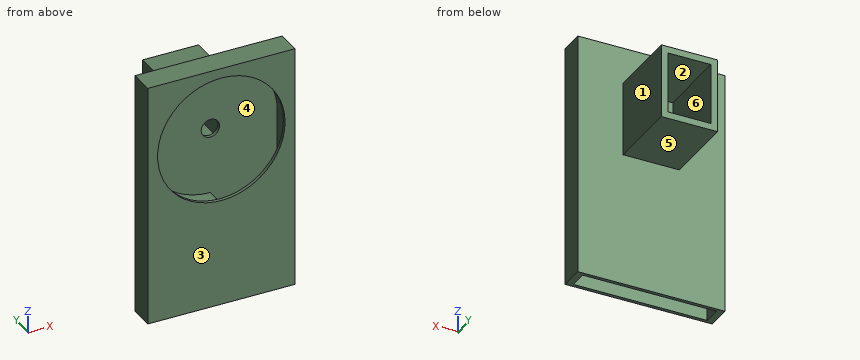
Autodesk Inventor part; units mm, degrees
ref_plane "YZ Plane" through (0, 0, 0) normal (1, 0, 0) x (0, 1, 0)
ref_plane "XZ Plane" through (0, 0, 0) normal (0, 1, 0) x (-1, 0, 0)
ref_plane "XY Plane" through (0, 0, 0) normal (0, 0, 1) x (1, 0, 0)
sketch "Sketch1" plane through (0, 0, 0) normal (0, 0, 1) x (1, 0, 0)
  line L0 (0, 0) -> (38.1, 0)
  line L1 (38.1, 0) -> (38.1, 6.35)
  line L2 (38.1, 6.35) -> (0, 6.35)
  line L3 (0, 6.35) -> (0, 0)
  line L4 (1.7272, 5.4864) -> (36.3728, 5.4864)
  line L5 (36.3728, 5.4864) -> (36.3728, 0.8636)
  line L6 (36.3728, 0.8636) -> (1.7272, 0.8636)
  line L7 (1.7272, 0.8636) -> (1.7272, 5.4864)
  dimension "d0" = 38.1
  dimension "d1" = 6.35
  dimension "d2" = 0.8636
  dimension "d3" = 1.7272
  dimension "d4" = 0.8636
  dimension "d5" = 1.7272
extrude "Extrusion1" add sketch "Sketch1" along normal blind 63.5
sketch "Sketch2" plane through (0, 0, 0) normal (0, -1, 0) x (1, 0, 0)
  line L0 (0, 63.5) -> (38.1, 63.5)
  circle A0 centre (19.05, 44.45) radius 16.51
  point P0 (0, 0)
  point P1 (19.05, 63.5)
  point P2 (19.05, 63.5)
  dimension "d8" = 33.02
  dimension "d9" = 19.05
extrude "Extrusion2" cut sketch "Sketch2" against normal up to next
sketch "Sketch3" plane through (1.7272, 5.4864, 0) normal (0, -1, 0) x (1, 0, 0)
  circle A0 centre (17.3228, 44.45) radius 16.51 construction
  line L0 (36.3728, 63.5) -> (-1.7272, 63.5) construction
  arc A1 (0, 44.45) -> (17.3228, 27.1272) centre (17.3228, 44.45) ccw
  line L1 (17.3228, 44.45) -> (0, 44.45) construction
  line L2 (17.3228, 44.45) -> (34.6456, 44.45) construction
  line L3 (17.3228, 44.45) -> (17.3228, 27.1272) construction
  line L4 (-1.7272, 0) -> (-1.7272, 63.5)
  arc A2 (17.3228, 27.1272) -> (0, 9.8044) centre (17.3228, 9.8044) ccw
  line L5 (17.3228, 9.8044) -> (0, 9.8044) construction
  line L6 (17.3228, 9.8044) -> (17.3228, 27.1272) construction
  arc A3 (34.6456, 44.45) -> (0, 44.45) centre (17.3228, 44.45) ccw
  line L7 (34.6456, 44.45) -> (34.6456, 61.7728)
  line L8 (34.6456, 61.7728) -> (0, 61.7728)
  line L9 (0, 61.7728) -> (0, 9.8044)
  point P0 (17.3228, 63.5)
  point P1 (17.3228, 61.7728)
  dimension "d12" = 33.02
  dimension "d13" = 19.05
  dimension "d14" = 180
  dimension "d15" = 90
  dimension "d16" = 1.7272
  dimension "d17" = 90
  dimension "d19" = 1.7272
  dimension "d20" = 19.05
extrude "Extrusion4" add sketch "Sketch3" along normal up to next contours L8 L7 A3
sketch "Sketch5" plane through (1.7272, 5.4864, 63.5) normal (0, -1, 0) x (1, 0, 0)
  arc A0 (17.3228, -1.7272) -> (0, -19.05) centre (17.3228, -19.05) ccw
  line L0 (17.3228, -19.05) -> (0, -19.05) construction
  line L1 (17.3228, -19.05) -> (17.3228, -1.7272) construction
  line L2 (36.3728, 0) -> (-1.7272, 0) construction
  line L3 (-1.7272, -63.5) -> (-1.7272, 0) construction
  line L4 (17.3228, -1.7272) -> (0, -1.7272)
  line L5 (0, -1.7272) -> (0, -19.05)
  point P0 (17.3228, 0)
  dimension "d35" = 90
  dimension "d36" = 1.7272
  dimension "d37" = 1.7272
extrude "Extrusion5" add sketch "Sketch5" along normal up to next
sketch "Sketch6" plane through (1.7272, 5.4864, 0) normal (0, -1, 0) x (1, 0, 0)
  arc A0 (0, 44.45) -> (17.3228, 27.1272) centre (17.3228, 44.45) ccw
  line L0 (17.3228, 44.45) -> (17.3228, 27.1272) construction
  line L1 (17.3228, 44.45) -> (0, 44.45) construction
  line L2 (36.3728, 63.5) -> (-1.7272, 63.5)
  line L3 (-1.7272, 0) -> (-1.7272, 63.5)
  line L4 (17.3228, 9.8044) -> (0, 9.8044) construction
  line L5 (17.3228, 9.8044) -> (17.3228, 27.1272) construction
  line L6 (0, 44.45) -> (0, 9.8044)
  line L7 (17.3228, 27.1272) -> (0, 9.8044)
  point P0 (17.3228, 63.5)
  dimension "d40" = 90
  dimension "d41" = 1.7272
  dimension "d42" = 19.05
  dimension "d43" = 90
  dimension "d44" = 1.7272
  dimension "d45" = 17.3228
extrude "Extrusion6" add sketch "Sketch6" along normal up to next
sketch "Sketch7" plane through (1.7272, 5.4864, 61.7728) normal (0, 0, 1) x (1, 0, 0)
  line L0 (17.3228, -4.6228) -> (0, -4.6228)
  line L1 (17.3228, 0) -> (34.6456, 0)
  line L2 (0, -4.6228) -> (34.6456, -4.6228)
  line L3 (34.6456, -4.6228) -> (34.6456, 0)
  line L4 (34.6456, 0) -> (0, 0)
  line L5 (0, 0) -> (0, -4.6228)
  point P0 (-1.7272, -5.4864)
extrude "Extrusion7" add sketch "Sketch7" along normal blind 1.7272
sketch "Sketch8" plane through (0, 6.35, 0) normal (0, 1, 0) x (1, 0, 0)
  line L0 (38.1, -63.5) -> (0, -63.5)
  line L1 (13.4938, -52.3875) -> (24.6062, -52.3875)
  line L2 (24.6062, -52.3875) -> (24.6062, -36.5125)
  line L3 (24.6062, -36.5125) -> (13.4938, -36.5125)
  line L4 (13.4938, -36.5125) -> (13.4938, -52.3875)
  line L5 (11.7666, -54.1147) -> (26.3335, -54.1147)
  line L6 (26.3335, -54.1147) -> (26.3335, -34.7853)
  line L7 (26.3335, -34.7853) -> (11.7665, -34.7853)
  line L8 (11.7665, -34.7853) -> (11.7666, -54.1147)
  point P0 (0, 0)
  point P1 (19.05, -44.45)
  point P2 (19.05, -63.5)
  point P3 (19.05, -36.5125)
  point P4 (13.4937, -44.45)
  dimension "d50" = 19.05
  dimension "d51" = 11.1125
  dimension "d52" = 15.875
  dimension "d53" = 1.7272
  dimension "d54" = 1.7272
  dimension "d55" = 1.7272
  dimension "d56" = 1.7272
extrude "Extrusion8" add sketch "Sketch8" along normal blind 19.05
sketch "Sketch9" plane through (0, 6.35, 0) normal (0, 1, 0) x (1, 0, 0)
  line L0 (38.1, -63.5) -> (0, -63.5)
  line L1 (13.4938, -52.3875) -> (13.4938, -36.5125)
  point P0 (0, 0)
  point P1 (19.05, -44.45)
  point P2 (19.05, -63.5)
  point P3 (13.4938, -44.45)
hole "Hole1" at (19.05, 6.35, 44.45) direction (0, -1, 0) diameter 4.7625 end through all
properties part number "main_chassis"
Geometry: final body of the model. Coordinates: model frame, mm. Face numbers are marked on the shaded views. A direction names the side the tool comes from. Give positions to 0.01 mm unless a question says otherwise; leave off trailing zeros. Order: outer loops, then holes, each group sorted by start corner. A loop starts at its lowest first (then second) coordinate and runs counter-clockwise, first axis right, second up. Notation, with made-up numbers: (-16, 6) -> (14, 6) arc R33 ccw to (14, 45) -> close; hole circle Ø10 at (-16, 13.5). An arc over 180 degrees is marked (long way). Answer as a JSON object with one key per item and string values.
Q1. Section B-B (y = 4.5). Output: boundary loops of the cut face in (x, z), plus the area to 3 significant figures.
Entries:
{"outline": "(0, 0) -> (1.73, 0) -> (1.73, 9.8) -> (19.05, 27.13) arc R17.32 cw (long way) to (36.37, 44.45) -> (36.37, 0) -> (38.1, 0) -> (38.1, 63.5) -> (0, 63.5) -> close", "area": "622 mm^2"}
Q2. First-contact query: pin 1 (1 mm diameter, centred on x = 20, y = 16.5, fed in from -Z); pin 2 (9.5 mm diameter, centred on y = 15, z = 45, fed in from -X); pin 3 (4 mm diameter, centred on x = 19.05, z = 44.45, fed in from -Y) (3 decimals); pin 4 (2 mm diameter, centred on x = 26.5, y = 21.5, fed in from +Z). Flat tips, straight axial feed; report the tip coordinate or a pass-through.
Entries:
{"pin 1": "stops at z = 34.79", "pin 2": "stops at x = 11.77", "pin 3": "passes through", "pin 4": "stops at z = 54.11"}
Q3. Material intervals for probe 1 along Y at (x, z) = (4.5, 11.5); probe 2 along X at (y, z) = (4.4, 44.45); probe 3 along Z at (x, y) = (19.05, 6.1), sorted ascending.
Entries:
{"probe 1": "y = 0 to 0.86, 5.49 to 6.35", "probe 2": "x = 0 to 1.73, 36.37 to 38.1", "probe 3": "z = 0 to 42.07, 46.83 to 63.5"}
Q4. Section C-C (x = 31.5). Output: boundary loops of the cut face in (y, z).
Entries:
{"outline": "(0, 0) -> (0.86, 0) -> (0.86, 33.61) -> (0, 33.61) -> close; (0, 55.29) -> (0.86, 55.29) -> (0.86, 56.49) -> (5.49, 56.49) -> (5.49, 0) -> (6.35, 0) -> (6.35, 63.5) -> (0, 63.5) -> close"}
Q5. Draft query along Z for the marked faces 3, 4, 5 and 6. Return one class per face: released by +Z, released by -Z, zero draft, split by the parting line, or undercut.
Entries:
{"face 3": "zero draft", "face 4": "undercut", "face 5": "released by -Z", "face 6": "undercut"}
Q6. Section D-D (z = 17). Output: boundary loops of the cut face in (x, y), plus the area to 3 significant figures.
Entries:
{"outline": "(0, 0) -> (38.1, 0) -> (38.1, 6.35) -> (0, 6.35) -> close; hole (8.92, 0.86) -> (36.37, 0.86) -> (36.37, 5.49) -> (8.92, 5.49) -> close", "area": "115 mm^2"}
Q7. Access query for the marked faces 1 and 2. Directions: +Z, -Z, +X, -X, +Y, -Y. A direction counts if a zero-diameter tool reaches every point of the face in a straight line with its end or side. Return the directions, or none.
Entries:
{"face 1": "+Z, -Z, +X, +Y", "face 2": "+Y"}
Q8. Section A-A (y = 9.25). Output: boundary loops of the cut face in (x, z), plus the area to 3 significant figures.
Entries:
{"outline": "(11.77, 34.79) -> (26.33, 34.79) -> (26.33, 54.11) -> (11.77, 54.11) -> close; hole (13.49, 36.51) -> (24.61, 36.51) -> (24.61, 52.39) -> (13.49, 52.39) -> close", "area": "105 mm^2"}
